Read the model definition and answer for the solid it produces. Units are mm, in the model's axes. Face numbers are marked on the shaded views. A direction names the side the tool comes from. Give positions to 0.01 mm unless a question says otherwise; leave off trailing zeros. Loops run counter-clockwise (first coordinate to the right, second up) from the corner with the lowest first, then second, coordinate; pieces in that order, holes last. Notation, with made-up numbers: (-9.75, 60) - (35.25, 60) arc R18 cw to (35.25, 86) - close; hole circle Ø1 at (-28, -30). An arc over 180 degrees is marked (long way). Use a Markdown table: item, result. Add a question column.
Item 1: A cutting plane is placed at C-C (y = 3). Determine the outline of the cut face in (x, z).
Item 2: A cutting plane is placed at D-D (z = 16.75). Determine the outline of the cut face in (x, y), plus the area to 3 significant figures.
Item 3: For a pull along Z with two mould halves and no side action, classify the marked faces 5, 6, 7 and 8 as +Z half, -Z half, draft (parallel to the pull), parting line (faces both ways), or undercut.
Item 4: A cutting plane is placed at B-B (x = 1.5). Determine the outline of the cut face in (y, z).
Item 5: Consider probe 1 along Z at (x, y) = (5.5, 2); probe 2 along Y at (x, z) = (15.5, 15.5). Determine where each line is inside the solid, lowest interval first. Write a range as [from, to].
Item 6: Each of these flat-tipped pins is pushed along its axis until it touches: P1, Ø3, axis at x = 3, y = -2.5, coming from the +Z side; P2, Ø12, axis at x = 11.5, z = 16, coming from the +Y side; P3, Ø4, axis at y = 2.5, z = 11, coming from the +X side; P4, Ø2, axis at y = 7.5, z = 8.5, coming from the -X side. Where does it stop, or does it pass through?
Item 7: Which of the six approach directions +Z, -Z, +X, -X, +Y, -Y give full straight-line access (tool end or side, diameter ignored) to the marked faces 1, 2, 3 and 4?
Item 8: A cutting plane is placed at A-A (x = 17). Determine the outline of the cut face in (y, z).
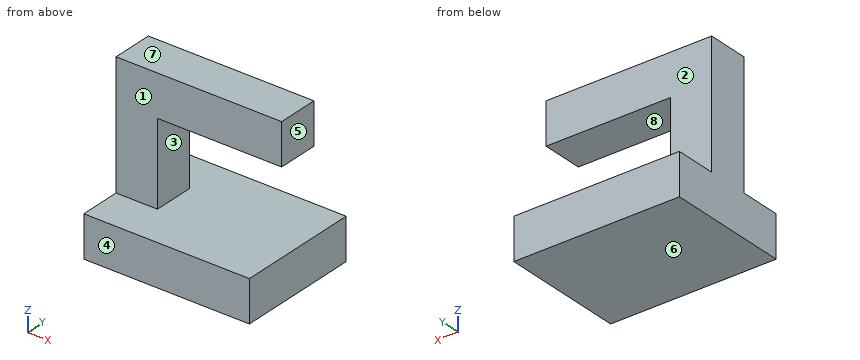
from build123d import *

# Parameters (mm, degrees)
BOX001_W     = 5
BOX001_H     = 5
BOX001_DEPTH = 20
BOX002_W     = 20
BOX002_H     = 5
BOX002_DEPTH = 5
BOX_W        = 20
BOX_H        = 15
BOX_DEPTH    = 5


with BuildPart() as cube001:
    # Box001 → Box001 (new body)
    with BuildSketch(Plane.XY):
        with Locations((2.5, 2.5)):
            Rectangle(BOX001_W, BOX001_H)
    extrude(amount=BOX001_DEPTH)


with BuildPart() as cube002:
    # Box002 → Box002 (new body)
    with BuildSketch(Plane.XY.offset(15)):
        with Locations((10, 2.5)):
            Rectangle(BOX002_W, BOX002_H)
    extrude(amount=BOX002_DEPTH)


with BuildPart() as fusion:
    # Box → Box (new body)
    with BuildSketch(Plane(origin=(0, -5, 0), x_dir=(1, 0, 0), z_dir=(0, 0, 1))):
        with Locations((10, 7.5)):
            Rectangle(BOX_W, BOX_H)
    extrude(amount=BOX_DEPTH)

    # Fusion: union Cube001, Cube002
    add(cube001.part)
    add(cube002.part)


solid = fusion.part
Geometry says:
| question | item | result |
|---|---|---|
| 1 | outline | (0, 0) - (20, 0) - (20, 5) - (5, 5) - (5, 15) - (20, 15) - (20, 20) - (0, 20) - close |
| 2 | outline | (0, 0) - (20, 0) - (20, 5) - (0, 5) - close |
| 2 | area | 100 mm² |
| 3 | face 5 | draft |
| 3 | face 6 | -Z half |
| 3 | face 7 | +Z half |
| 3 | face 8 | undercut |
| 4 | outline | (-5, 0) - (10, 0) - (10, 5) - (5, 5) - (5, 20) - (0, 20) - (0, 5) - (-5, 5) - close |
| 5 | probe 1 | [0, 5], [15, 20] |
| 5 | probe 2 | [0, 5] |
| 6 | P1 | z = 5 |
| 6 | P2 | y = 5 |
| 6 | P3 | x = 5 |
| 6 | P4 | through |
| 7 | face 1 | +Z, +X, -X, -Y |
| 7 | face 2 | +Z, +X, -X, +Y |
| 7 | face 3 | +X, +Y, -Y |
| 7 | face 4 | +Z, -Z, +X, -X, -Y |
| 8 | outline | (-5, 0) - (10, 0) - (10, 5) - (-5, 5) - close; (0, 15) - (5, 15) - (5, 20) - (0, 20) - close |
